Verification items for the finished model (mm, model axes). A direction names the side the tool comes from. Round coordinates to 2 decimals unless told otherwise and drop trailing zeros. Write each loop counter-clockwise with the first axis right and the second up, starting at its lowest first coordinate (ties: lowest second). Pieces come first, ordered by that corner, then holes. Notation, with made-up numbers: (-15, 86.25) -> (21, 86.25) arc R16 ccw to (21, 93.25) -> close; hole circle Ø3 at (18.25, 36.5). An arc over 180 degrees is marked (long way). Answer as a JSON object with one key per item and string values. Group by question number.
(1) Scan lines: L1, parallel to Y at x = 0.5, z = -2.5; L2, parallel to Y at x = 76.1, z = -1.9; L3, parallel to X at y = -3.5, z = -2.6. Record each from-to range of solid material in increasing order. Write a range as from..to.
(2) Draft check along Y on faces 3 (the face through (90, -6.25, -2)), 4 (the face through (46, 0, -5)), 5 (the face through (-0.419, -8.016, -2.465)), 6 (the face through (110, 0, -3)). Enter one of: released by +Y, released by -Y, zero draft, split by the parting line, or undercut.
(3) Sectioned sample at B-B on z = -1.05. Count the separate pieces of the cut face and the enclosed holes in it, and give its area (3 significant figures).
(4) Sectioned sample at C-C on y = 11.5. Record the cut outline in (x, z).
(5) Set-up check for faces 1 (the face through (46, -20, -3)), 2 (the face through (78.75, 0, -2)): record each of +Z, -Z, +X, -X, +Y, -Y from which the full face is reachable in a straight line by a thin tool's end or side.
(6) Gauge pin test, flat ends, axial feed: pin 1 Ø3 at (y, z) = (-7.5, -4) entering from -X; pin 2 Ø2 at (y, z) = (-15.5, -2.5) entering from -X (3 decimals); pin 3 Ø2.5 at (y, z) = (2.5, -2.5) entering from +X. Record the tip position at first contact, or that the pin passes through.
(7) Sectioned sample at A-A on x = 86. Record the cut outline in (y, z), and give its area (4 significant figures).
```python
from build123d import *

# Parameters (mm, degrees)
BOSS_EXTRUDE1_DEPTH   = 5
CUT_EXTRUDE1_REACH    = 113.915
SKETCH2_R             = 1.5
SKETCH2_R_2           = 1.1
BODY_MOVE_COPY1_ANGLE = 90
SKETCH19_R            = 1.05
SKETCH19_W            = 22.5
SKETCH19_H            = 12.5
CUT_EXTRUDE9_DEPTH    = 112.915146428


with BuildPart() as part:
    # Sketch1 → Boss-Extrude1 (new body)
    with BuildSketch(Plane(origin=(0, 0, 0), x_dir=(1, 0, 0), z_dir=(0, 1, 0))):
        with BuildLine():
            Line((90, -20), (0, -20))
            ThreePointArc((0, -20), (-20, 0), (0, 20))
            Line((0, 20), (90, 20))
            ThreePointArc((90, 20), (110, 0), (90, -20))
        make_face()
    extrude(amount=BOSS_EXTRUDE1_DEPTH)

    # Sketch2 → Cut-Extrude1 (cut, up to next)
    with BuildSketch(Plane(origin=(0, 5, 0), x_dir=(1, 0, 0), z_dir=(0, 1, 0)), mode=Mode.PRIVATE) as cut_extrude1_sk1:
        with Locations(Location((0, 0, 0), (0, 0, 270))):
            Circle(SKETCH2_R)
    cut_extrude1_tool1 = extrude(cut_extrude1_sk1.sketch, amount=-CUT_EXTRUDE1_REACH, mode=Mode.PRIVATE) & part.part
    # Sketch2 → Cut-Extrude1 (cut, up to next)
    with BuildSketch(Plane(origin=(0, 5, 0), x_dir=(1, 0, 0), z_dir=(0, 1, 0)), mode=Mode.PRIVATE) as cut_extrude1_sk2:
        with Locations(Location((0, 7, 0), (0, 0, 270))):
            Circle(SKETCH2_R_2)
    cut_extrude1_tool2 = extrude(cut_extrude1_sk2.sketch, amount=-CUT_EXTRUDE1_REACH, mode=Mode.PRIVATE) & part.part
    # Sketch2 → Cut-Extrude1 (cut, up to next)
    with BuildSketch(Plane(origin=(0, 5, 0), x_dir=(1, 0, 0), z_dir=(0, 1, 0)), mode=Mode.PRIVATE) as cut_extrude1_sk3:
        with Locations(Location((7.001, 0.001, 0), (0, 0, 270))):
            Circle(SKETCH2_R_2)
    cut_extrude1_tool3 = extrude(cut_extrude1_sk3.sketch, amount=-CUT_EXTRUDE1_REACH, mode=Mode.PRIVATE) & part.part
    # Sketch2 → Cut-Extrude1 (cut, up to next)
    with BuildSketch(Plane(origin=(0, 5, 0), x_dir=(1, 0, 0), z_dir=(0, 1, 0)), mode=Mode.PRIVATE) as cut_extrude1_sk4:
        with Locations(Location((0.002, -7, 0), (0, 0, 270))):
            Circle(SKETCH2_R_2)
    cut_extrude1_tool4 = extrude(cut_extrude1_sk4.sketch, amount=-CUT_EXTRUDE1_REACH, mode=Mode.PRIVATE) & part.part
    # Sketch2 → Cut-Extrude1 (cut, up to next)
    with BuildSketch(Plane(origin=(0, 5, 0), x_dir=(1, 0, 0), z_dir=(0, 1, 0)), mode=Mode.PRIVATE) as cut_extrude1_sk5:
        with Locations(Location((-6.999, -0.001, 0), (0, 0, 270))):
            Circle(SKETCH2_R_2)
    cut_extrude1_tool5 = extrude(cut_extrude1_sk5.sketch, amount=-CUT_EXTRUDE1_REACH, mode=Mode.PRIVATE) & part.part
    add(cut_extrude1_tool1.solids().sort_by_distance((0, 5, 0))[0], mode=Mode.SUBTRACT)
    add(cut_extrude1_tool2.solids().sort_by_distance((0, 5, -7))[0], mode=Mode.SUBTRACT)
    add(cut_extrude1_tool3.solids().sort_by_distance((7.001, 5, -0.001))[0], mode=Mode.SUBTRACT)
    add(cut_extrude1_tool4.solids().sort_by_distance((0.002, 5, 7))[0], mode=Mode.SUBTRACT)
    add(cut_extrude1_tool5.solids().sort_by_distance((-6.999, 5, 0.001))[0], mode=Mode.SUBTRACT)


with BuildPart() as part_1:
    # Body-Move/Copy1: moved
    add(part.part.rotate(Axis((0, 0, 0), (1, 0, 0)), BODY_MOVE_COPY1_ANGLE))

    # Sketch19 → Cut-Extrude9 (cut, through all)
    with BuildSketch(Plane.XY.offset(5)):
        with Locations((103.9, 0)):
            Circle(SKETCH19_R)
        with Locations(Location((76.1, 0, 0), (0, 0, 180))):
            Circle(SKETCH19_R)
        with Locations((90, 0)):
            Rectangle(SKETCH19_W, SKETCH19_H)
    extrude(amount=-CUT_EXTRUDE9_DEPTH, mode=Mode.SUBTRACT)


with BuildPart() as part_2:
    # Body-Move/Copy2: moved
    add(part_1.part.moved(Location((0, 0, -5))))


solid = part_2.part
```
Computed values:
{
 "1": {"L1": "-20..-7.98, -6.02..-1.41, 1.41..6.02, 7.98..20", "L2": "-20..-1.05, 1.05..20", "L3": "-19.69..78.75, 101.25..109.69"},
 "2": {"face 3": "undercut", "face 4": "zero draft", "face 5": "undercut", "face 6": "split by the parting line"},
 "3": {"separate pieces": "1", "enclosed holes": "8", "area": "4,550 mm2"},
 "4": {"outline": "(-16.36, -5) -> (106.36, -5) -> (106.36, 0) -> (-16.36, 0) -> close"},
 "5": {"face 1": "+Z, -Z, +X, -X, -Y", "face 2": "+Z, -Z"},
 "6": {"pin 1": "x = -19.08", "pin 2": "x = -13.775", "pin 3": "x = 109.96"},
 "7": {"outline": "(-20, -5) -> (-6.25, -5) -> (-6.25, 0) -> (-20, 0) -> close; (6.25, -5) -> (20, -5) -> (20, 0) -> (6.25, 0) -> close", "area": "137.5 mm2"}
}
